from build123d import *

# Parameters (mm, degrees)
F1_DEPTH = 82.55
F2_R     = 17.4625
F3_DEPTH = 12.7
F5_DEPTH = 25.4
F6_R     = 17.4625
F7_DEPTH = 25.4


with BuildPart() as f1:
    # F0 (on Front) → F1 (new body)
    with BuildSketch(Plane.XZ):
        Polygon((0, 116.06285), (0, 0), (190.5, 0), (190.5, 12.7), (25.4, 12.7), (25.4, 116.06285), align=None)
    extrude(amount=F1_DEPTH)

    # F2 (on face) → F3 (cut)
    with BuildSketch(Plane.XY.offset(12.7)):
        with Locations((76.2, -41.275)):
            Circle(F2_R)
        with Locations((152.4, -41.275)):
            Circle(F2_R)
    extrude(amount=-F3_DEPTH, mode=Mode.SUBTRACT)

    # F4 (on face) → F5 (cut)
    with BuildSketch(Plane(origin=(0, 0, 0), x_dir=(0, -1, 0), z_dir=(-1, 0, 0))):
        with BuildLine():
            ThreePointArc((0, 58.031425), (41.275, 99.306425), (82.55, 58.031425))
            Line((82.55, 58.031425), (82.55, 116.06285))
            Line((82.55, 116.06285), (0, 116.06285))
            Line((0, 116.06285), (0, 58.031425))
        make_face()
    extrude(amount=-F5_DEPTH, mode=Mode.SUBTRACT)

    # F6 (on face) → F7 (cut)
    with BuildSketch(Plane.YZ.offset(25.4)):
        with Locations((-41.275, 58.031425)):
            Circle(F6_R)
    extrude(amount=-F7_DEPTH, mode=Mode.SUBTRACT)


solid = f1.part
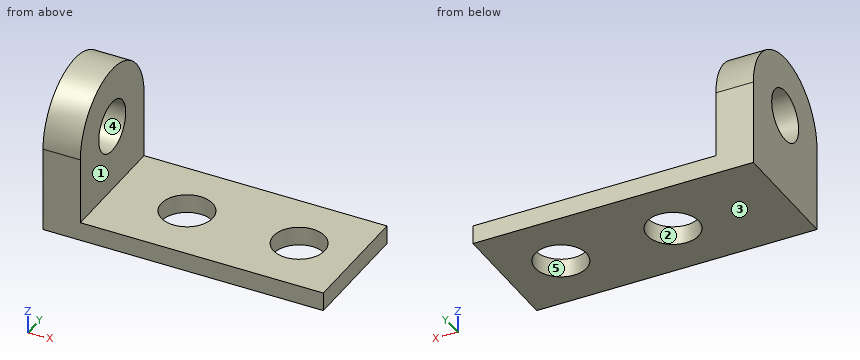
The model under review builds one solid part; all positions refer to its coordinate system, in mm. Face numbers are marked on the shaded views. A direction names the side the tool comes from. Coordinates: 2 decimals unless noted, no trailing zeros. Loops run counter-clockwise (first coordinate to the right, second up) from the corner with the lowest first, then second, coordinate; pieces in that order, holes last. Notation, with made-up numbers: M 67,-19 L 88,-19 A13 cw 88,4 Z; hole C 68,-30 d9. An arc over 180 degrees is marked long. Put each result on its own line as item: value. Start each with the question number.
Q1. The part is to be moulded in two halves that separate along Z. For the marked faces 3, 4 and 5, say which applies: +Z half, -Z half, draft (parallel to the pull), parting line (faces both ways), or undercut.
Q2. Add section A-A (x = 152.4). Write out the cut boundary in (y, z).
Q3. Add section D-D (y = -9). Write out the cut boundary in (x, z), and give its area (3 significant figures).
Q4. Clearance check with flat-ended pins moving along their axes: pin 1 (6 mm diameter, centred on x = 108, y = -13.5, fed in from +Z); pin 2 (3 mm diameter, centred on y = -70.5, z = 31, fed in from +X). State where each tip first meets the part, or that it passes through.
Q5. For the marked faces 1 and 2, list the 3-axis set-ups (+Z, -Z, +X, -X, +Y, -Y) from which the entire face can be reached by the end or side of a thin tool; tool diameter is ignored.
Q6. Add section B-B (y = -31). Write out the cut boundary in (x, z), and give its area (3 significant figures).
Q7. Add section C-C (z = 63.5). Write out the cut boundary in (x, y).
Q8. Wall thickness on line 1 (Y direction, x = 10, z = 58.5); line 2 (Z direction, x = 117, y = -20.5); line 3 (Y direction, x = 76.2, z = 9): over which ranges is each line inside the solid? List them lowest first.
Answers:
1. face 3: -Z half
1. face 4: undercut
1. face 5: draft
2. outline: M -82.55,0 L -58.74,0 L -58.74,12.7 L -82.55,12.7 Z; M -23.81,0 L 0,0 L 0,12.7 L -23.81,12.7 Z
3. outline: M 0,0 L 190.5,0 L 190.5,12.7 L 25.4,12.7 L 25.4,83.76 L 0,83.76 Z
3. area: 4,220 mm^2
4. pin 1: stops at z = 12.7
4. pin 2: stops at x = 25.4
5. face 1: +Z, +X, +Y, -Y
5. face 2: +Z, -Z
6. outline: M 0,0 L 62.08,0 L 62.08,12.7 L 25.4,12.7 L 25.4,43.91 L 0,43.91 Z; M 0,72.15 L 25.4,72.15 L 25.4,98.01 L 0,98.01 Z; M 90.32,0 L 138.28,0 L 138.28,12.7 L 90.32,12.7 Z; M 166.52,0 L 190.5,0 L 190.5,12.7 L 166.52,12.7 Z
6. area: 3,150 mm^2
7. outline: M 0,-82.19 L 25.4,-82.19 L 25.4,-57.86 L 0,-57.86 Z; M 0,-24.69 L 25.4,-24.69 L 25.4,-0.36 L 0,-0.36 Z
8. line 1: y = -82.55 to -58.73, -23.82 to 0
8. line 2: z = 0 to 12.7
8. line 3: y = -82.55 to -58.74, -23.81 to 0
